from build123d import *

# Parameters (mm, degrees)
BOSS_EXTRUDE1_DEPTH              = 6.35
F_21_64_0_32813_DIAMETER_HOLE1_D = 8.334502
LPATTERN1_COUNT                  = 2
LPATTERN1_PITCH                  = 38.1
LPATTERN1_COUNT_DIR2             = 2
LPATTERN1_PITCH_DIR2             = 38.1
F_21_64_0_32813_DIAMETER_HOLE2_D = 8.334502
LPATTERN2_COUNT                  = 2
LPATTERN2_PITCH                  = 38.1
LPATTERN2_COUNT_DIR2             = 3
LPATTERN2_PITCH_DIR2             = 38.1
F_21_64_0_32813_DIAMETER_HOLE3_D = 8.334502
LPATTERN3_COUNT                  = 2
LPATTERN3_PITCH                  = 38.1
LPATTERN3_COUNT_DIR2             = 3
LPATTERN3_PITCH_DIR2             = 38.1
FILLET1_R                        = 6.35


with BuildPart() as part:
    # Sketch1 → Boss-Extrude1 (new body)
    with BuildSketch(Plane.XY):
        Polygon((0, 0), (76.2, 0), (76.2, -76.2), (167.256744728, -198.406502444), (106.153493506, -243.934874808), (38.1, -152.600845184), (-29.953493506, -243.934874808), (-91.056744728, -198.406502444), (0, -76.2), align=None)
    extrude(amount=BOSS_EXTRUDE1_DEPTH)

    # 21/64 (0.32813) Diameter Hole1 (through all)
    with Locations(Plane.XY.offset(6.35)):
        with Locations((57.15, -19.05)):
            f_21_64_0_32813_diameter_hole1 = Hole(F_21_64_0_32813_DIAMETER_HOLE1_D / 2)

    # LPattern1: 21_64 _0.32813_ Diameter Hole1 2 × 2
    with Locations(*[(-i * LPATTERN1_PITCH, -j * LPATTERN1_PITCH_DIR2, 0) for i in range(LPATTERN1_COUNT) for j in range(LPATTERN1_COUNT_DIR2) if (i, j) != (0, 0)]):
        add(f_21_64_0_32813_diameter_hole1, mode=Mode.SUBTRACT)

    # 21/64 (0.32813) Diameter Hole2 (through all)
    with Locations(Plane.XY.offset(6.35)):
        with Locations((-64.398838831, -194.512782729)):
            f_21_64_0_32813_diameter_hole2 = Hole(F_21_64_0_32813_DIAMETER_HOLE2_D / 2)

    # LPattern2: 21_64 _0.32813_ Diameter Hole2 2 × 3
    with Locations(*[Vector(0.8018799372965569, -0.5974852016253374, 0) * (i * LPATTERN2_PITCH) + Vector(0.5974852016253378, 0.8018799372965567, 0) * (j * LPATTERN2_PITCH_DIR2) for i in range(LPATTERN2_COUNT) for j in range(LPATTERN2_COUNT_DIR2) if (i, j) != (0, 0)]):
        add(f_21_64_0_32813_diameter_hole2, mode=Mode.SUBTRACT)

    # 21/64 (0.32813) Diameter Hole3 (through all)
    with Locations(Plane.XY.offset(6.35)):
        with Locations((140.598838831, -194.512782729)):
            f_21_64_0_32813_diameter_hole3 = Hole(F_21_64_0_32813_DIAMETER_HOLE3_D / 2)

    # LPattern3: 21_64 _0.32813_ Diameter Hole3 2 × 3
    with Locations(*[Vector(-0.8018799372965564, -0.597485201625338, 0) * (i * LPATTERN3_PITCH) + Vector(-0.5974852016253386, 0.8018799372965559, 0) * (j * LPATTERN3_PITCH_DIR2) for i in range(LPATTERN3_COUNT) for j in range(LPATTERN3_COUNT_DIR2) if (i, j) != (0, 0)]):
        add(f_21_64_0_32813_diameter_hole3, mode=Mode.SUBTRACT)

    # Fillet1
    fillet1_edges = [part.edges().sort_by_distance(p)[0] for p in [
        (38.1, -152.600845184, 3.175),
    ]]
    fillet(fillet1_edges, radius=FILLET1_R)


solid = part.part
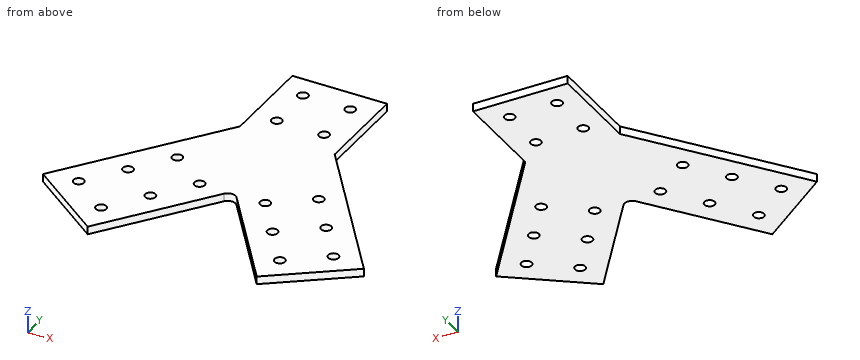
Can you work these out from the model? Positions are in its coordinate system, mm. Coordinates: 2 decimals unless noted, no trailing zeros. Write each loop counter-clockwise with the first axis right and the second up, starting at its lowest first coordinate (ties: lowest second). Pieces come first, ordered by that corner, then holes. Notation, with made-up numbers: (28.5, 28.5) -> (81.5, 28.5) arc R10 ccw to (81.5, 47.5) -> close; hole circle Ø8 at (-16, -16.5). An arc over 180 degrees is marked (long way). Answer as CSV lines item,"result".
1) If we section it at A-A on y = -19.05: Please give me the cut outline in (x, z).
Check result:
outline,"(0, 0) -> (14.88, 0) -> (14.88, 6.35) -> (0, 6.35) -> close; (23.22, 0) -> (52.98, 0) -> (52.98, 6.35) -> (23.22, 6.35) -> close; (61.32, 0) -> (76.2, 0) -> (76.2, 6.35) -> (61.32, 6.35) -> close"
2) If we section it at B-B on z = 3.5: Count the separate pieces of the cut face and the enclosed holes in it, then the cut area to 3 significant figures.
Check result:
separate pieces,"1"
enclosed holes,"16"
area,"28,200 mm²"
3) If we section it at C-C on x = 57.15: Please give me the cut outline in (y, z).
Check result:
outline,"(-178.17, 0) -> (-61.32, 0) -> (-61.32, 6.35) -> (-178.17, 6.35) -> close; (-52.98, 0) -> (-23.22, 0) -> (-23.22, 6.35) -> (-52.98, 6.35) -> close; (-14.88, 0) -> (0, 0) -> (0, 6.35) -> (-14.88, 6.35) -> close"
4) Will these pins go through, and if not, where does the flat tip stop? P1, Ø1, axis at y = -165, z = 5.5, coming from the +X side; P2, Ø1.5, axis at y = -158.5, z = 5, coming from the -X side; P3, Ø2, axis at x = 120.5, z = 4.5, coming from the -Y side.
Check result:
P1,"x = 142.74"
P2,"x = -61.88"
P3,"y = -233.99"
5) If we section it at D-D on y = -69: Please give me the cut outline in (x, z).
Check result:
outline,"(0, 0) -> (76.2, 0) -> (76.2, 6.35) -> (0, 6.35) -> close"
6) If I drill on line 1 (X direction, y = -167.5, z = 0.5); line 2 (X direction, y = -60, z = 6.25); line 3 (X direction, y = -136, z = 3.5), over which ranges is the centre line in solid material (lowest first)? Write a range as from..to.
Check result:
line 1,"-68.03..-43.84, -39.43..27, 49.2..115.63, 120.04..144.23"
line 2,"0..16.01, 22.09..54.11, 60.19..76.2"
line 3,"-44.56..-22.13, -15.61..91.81, 98.33..120.76"
